from build123d import *

# Parameters (mm, degrees)
BOSS_EXTRUDE1_DEPTH = 3
SKETCH3_R           = 2.5
CUT_EXTRUDE1_DEPTH  = 4


with BuildPart() as part:
    # Sketch1 → Boss-Extrude1 (new body)
    with BuildSketch(Plane.XY):
        Polygon((0, 186.26), (0, 438.1), (281.05, 438.1), (281.05, 186.26), (263.05, 186.26), (263.05, 131.26), (281.05, 131.26), (281.05, 0), (0, 0), (0, 131.26), (18, 131.26), (18, 186.26), align=None)
    extrude(amount=BOSS_EXTRUDE1_DEPTH)

    # Sketch3 → Cut-Extrude1 (cut, through all)
    with BuildSketch(Plane.XY.offset(3)):
        with Locations((65.525, 428.6)):
            Circle(SKETCH3_R)
        with Locations((115.525, 428.6)):
            Circle(SKETCH3_R)
        with Locations((15.525, 428.6)):
            Circle(SKETCH3_R)
        with Locations((265.525, 428.6)):
            Circle(SKETCH3_R)
        with Locations((165.525, 428.6)):
            Circle(SKETCH3_R)
        with Locations((215.525, 428.6)):
            Circle(SKETCH3_R)
        with Locations((215.525, 9.5)):
            Circle(SKETCH3_R)
        with Locations((165.525, 9.5)):
            Circle(SKETCH3_R)
        with Locations((265.525, 9.5)):
            Circle(SKETCH3_R)
        with Locations((15.525, 9.5)):
            Circle(SKETCH3_R)
        with Locations((115.525, 9.5)):
            Circle(SKETCH3_R)
        with Locations((65.525, 9.5)):
            Circle(SKETCH3_R)
        with Locations((9.5, 338.1)):
            Circle(SKETCH3_R)
        with Locations((9.5, 288.1)):
            Circle(SKETCH3_R)
        with Locations((9.5, 238.1)):
            Circle(SKETCH3_R)
        with Locations((9.5, 100)):
            Circle(SKETCH3_R)
        with Locations((271.55, 100)):
            Circle(SKETCH3_R)
        with Locations((271.55, 238.1)):
            Circle(SKETCH3_R)
        with Locations((271.55, 288.1)):
            Circle(SKETCH3_R)
        with Locations((271.55, 338.1)):
            Circle(SKETCH3_R)
    extrude(amount=-CUT_EXTRUDE1_DEPTH, mode=Mode.SUBTRACT)


solid = part.part
Can you work these out from the model? Positions are in its coordinate system, mm. Coordinates: 2 decimals unless noted, no trailing zeros. Put each result on its own line as item: value. Start each with the question number.
Item 1: For pin 1 (0.9 mm diameter, centred on y = 154.5, z = 1, fed in from +X), with a flat end and sliding along its axis, tell me the tip position at first contact or that it passes through.
Item 2: If I drill on line 1 along X through (y, z) = (238.1, 1.7); line 2 along Y through (x, z) = (271.55, 0.65); line 3 along X through (y, z) = (158, 2.25), over which ranges is the centre line in solid material (lowest first)?
Item 3: Suppose I cut it at A-A (z = 1.95). State how many separate pieces and enclosed holes the cut face has, and give its area (3 significant figures).
Here are the results:
1. pin 1: x = 263.05
2. line 1: 0 to 7, 12 to 269.05, 274.05 to 281.05
2. line 2: 0 to 97.5, 102.5 to 131.26, 186.26 to 235.6, 240.6 to 285.6, 290.6 to 335.6, 340.6 to 438.1
2. line 3: 18 to 263.05
3. separate pieces: 1
3. enclosed holes: 20
3. area: 121,000 mm²
